from build123d import *

# Parameters (mm, degrees)
F0_W     = 254
F0_H     = 25.4
F1_DEPTH = 13.97
F2_W     = 267.5041258335
F2_H     = 23.1854785234
F3_DEPTH = 12.7
F5_D     = 3.175
F7_D     = 3.175


with BuildPart() as f1:
    # F0 (on Front) → F1 (new body)
    with BuildSketch(Plane.XZ):
        with Locations((3.752566874, -11.3044876873)):
            Rectangle(F0_W, F0_H)
    extrude(amount=F1_DEPTH)

    # F2 (on Front) → F3 (cut)
    with BuildSketch(Plane.XZ):
        with Locations((1.6082376242, -11.5927392617)):
            Rectangle(F2_W, F2_H)
    extrude(amount=F3_DEPTH, mode=Mode.SUBTRACT)

    # F5 (through all)
    with Locations(Plane.XY.offset(1.3955123127)):
        with Locations((123.8327398896, -6.8190763704), (115.6149059534, -6.6323070787), (-116.3921877742, -7.0234532468), (-107.0919632912, -7.0234532468), (-98.6859947443, -7.0234532468), (-90.6377211213, -7.0234532468)):
            Hole(F5_D / 2)

    # F7 (through all)
    with Locations(Plane(origin=(0, 0, 0), x_dir=(1, 0, 0), z_dir=(0, 1, 0))):
        with Locations((121.5464174747, 6.637244951), (121.5464174747, 15.8025249839)):
            Hole(F7_D / 2)


solid = f1.part
The listing builds one solid part. Answer for the finished solid, in the listing's coordinates (mm). A direction names the side the tool comes from. Round coordinates to 2 decimals unless told otherwise and drop trailing zeros. Order: outer loops, then holes, each group sorted by start corner. A loop starts at its lowest first (then second) coordinate and runs counter-clockwise, first axis right, second up. Notation, with made-up numbers: (26, -35.5) -> (65, -35.5) arc R12 ccw to (65, -28.5) -> close; hole circle Ø10 at (66, 50). An arc over 180 degrees is marked (long way). Put each result on its own line as item: value.
Q1. Which of the six approach directions +Z, -Z, +X, -X, +Y, -Y give full straight-line access (tool end or side, diameter ignored) to faces 1 (the flat face through (2, -13.97, -11)), 2 (the flat face through (2, -12.7, -11))?
Results list:
face 1: +Z, -Z, +X, -X, -Y
face 2: +X, -X, +Y
Q2. Determine the mould class of faces 3 (the flat face through (2, -7, -24.004)), 4 (the flat face through (130.753, -13, -11)), 5 (the flat face through (2, -6, 0)), 6 (the flat face through (2, -6, -23.185)) for opening direction Z: pulls with the +Z half, pulls with the -Z half, needs draft (parallel to the pull), parting line crosses it, or undercut.
Results list:
face 3: pulls with the -Z half
face 4: needs draft
face 5: undercut
face 6: undercut
Q3. Consider line 1 along Z through (x, y) = (-93.5, -9.5); line 2 along Y through (x, z) = (11, -0.5). Determine where each line is inside the solid, lowest interval first.
Results list:
line 1: -24 to -23.19, 0 to 1.4
line 2: -13.97 to -12.7
Q4. Section A-A, the plane x = 9.5 is taken. Write down the section's boundary in (y, z).
Results list:
outline: (-13.97, -24) -> (0, -24) -> (0, -23.19) -> (-12.7, -23.19) -> (-12.7, 0) -> (0, 0) -> (0, 1.4) -> (-13.97, 1.4) -> close
Q5. This flat-tipped pin is pushed along its axis until it touches: P1, Ø2, axis at x = 53.5, z = -17.5, coming from the +Y side. Where does it stop, or does it pass through?
Results list:
P1: y = -12.7
